Autodesk Inventor part; units mm, degrees
ref_plane "YZ Plane" through (0, 0, 0) normal (1, 0, 0) x (0, 1, 0)
ref_plane "XZ Plane" through (0, 0, 0) normal (0, 1, 0) x (-1, 0, 0)
ref_plane "XY Plane" through (0, 0, 0) normal (0, 0, 1) x (1, 0, 0)
sketch "Skizze1" plane through (0, 0, 0) normal (0, 1, 0) x (-1, 0, 0)
  circle A0 centre (0, 0) radius 9.5
  circle A1 centre (0, 0) radius 11.5
  circle A2 centre (0, 0) radius 8.5
  circle A3 centre (0, 0) radius 3
  circle A4 centre (0, 0) radius 20
  line L0 (10.4225, 4.8601) -> (18.1262, 8.4524)
  line L1 (10.4225, -4.8601) -> (18.1262, -8.4524)
  line L2 (28, 0) -> (-28, 0)
  line L3 (-10.4225, 4.8601) -> (-18.1262, 8.4524)
  line L4 (-10.4225, -4.8601) -> (-18.1262, -8.4524)
  dimension "d0" = 19
  dimension "d1" = 23
  dimension "d2" = 17
  dimension "d3" = 6
  dimension "d8" = 40
  dimension "d10" = 50
extrude "Extrusion1" add sketch "Skizze1" along normal blind 2 contours L2 A2 A0 | L2 A1 A0 | A0 L2 A1 | A0 L2 A2 | L2 A4 L1 A1 | A1 L0 A4 L2 | L2 A3 A2 | A2 L2 A3 | L2 A4 L3 A1 | A1 L4 A4 L2
extrude "Extrusion2" add sketch "Skizze1" against normal blind 10 contours L2 A2 A0 | A0 L2 A2 | L2 A3 A2 | A2 L2 A3
sketch "Skizze2" plane through (0, 2, 0) normal (0, 1, 0) x (1, 0, 0)
  circle A0 centre (0, 0) radius 3
  arc A1 (-18.1262, 8.4524) -> (-18.1262, -8.4524) centre (0, 0) ccw
  line L0 (-2.8868, 5) -> (2.8868, 5)
  line L1 (2.8868, 5) -> (5.7735, 0)
  line L2 (5.7735, 0) -> (2.8868, -5)
  line L3 (2.8868, -5) -> (-2.8868, -5)
  line L4 (-2.8868, -5) -> (-5.7735, 0)
  line L5 (-5.7735, 0) -> (-2.8868, 5)
  dimension "d11" = 10
extrude "Extrusion3" cut sketch "Skizze2" against normal blind 4
properties part number "Unterdruckventil_Gegenhalter"
Verification items for the finished model (mm, model axes). A direction names the side the tool comes from. Give positions to 0.01 mm unless a question says otherwise; leave off trailing zeros. Order: outer loops, then holes, each group sorted by start corner. A loop starts at its lowest first (then second) coordinate and runs counter-clockwise, first axis right, second up. Notation, with made-up numbers: (88, -22.5) -> (142, -22.5) arc R22 cw to (142, -0.5) -> close; hole circle Ø3 at (72.5, -0.5). An arc over 180 degrees is marked (long way). One line per item, written item: value.
(1) Sectioned sample at A-A on x = 0. Record the cut outline in (y, z).
Final values:
outline: (-10, -9.5) -> (0, -9.5) -> (0, -11.5) -> (2, -11.5) -> (2, -5) -> (-2, -5) -> (-2, -3) -> (-10, -3) -> close; (-10, 3) -> (-2, 3) -> (-2, 5) -> (2, 5) -> (2, 11.5) -> (0, 11.5) -> (0, 9.5) -> (-10, 9.5) -> close
(2) Sectioned sample at D-D on z = -3.75. Record the cut outline in (x, y), then the cut area to 3 significant figures.
Final values:
outline: (-19.65, 0) -> (-8.73, 0) -> (-8.73, -10) -> (8.73, -10) -> (8.73, 0) -> (19.65, 0) -> (19.65, 2) -> (3.61, 2) -> (3.61, -2) -> (-3.61, -2) -> (-3.61, 2) -> (-19.65, 2) -> close
area: 224 mm^2
(3) Scan lines: line 1 along Z through (x, y) = (0, -4.5); line 2 along Y through (x, z) = (-5, 8.25); line 3 along Z through (x, y) = (2.5, 1.5). Record each from-to range of solid material in increasing order. Write a range as [from, to].
Final values:
line 1: [-9.5, -3], [3, 9.5]
line 2: [0, 2]
line 3: [-11.22, -5], [5, 11.22]
(4) Tool access check on faces 1 (the face through (0, 0, -10)), 2 (the face through (14.22, 0.99, -6.63)), 3 (the face through (0, 0, 5)). Record the directions out of +Z, -Z, +X, -X, +Y, -Y that give a thin tool (end or side, any length) a straight path to the whole face; none if there is none.
Final values:
face 1: -Y
face 2: -Z, +Y, -Y
face 3: +Y
(5) Gauge pin test, flat ends, axial feed: pin 1 (6 mm diameter, centred on y = 0, z = 8.5, fed in from -X); pin 2 (2 mm diameter, centred on y = -5, z = 4, fed in from +X); pin 3 (1.2 mm diameter, centred on x = 1.5, y = 1, fed in from -Z); pin 4 (2 mm diameter, centred on x = 0.5, y = 0.5, fed in from +Z). Record the tip position at first contact, or that the pin passes through.
Final values:
pin 1: x = -19.23
pin 2: x = 9.01
pin 3: z = -11.46
pin 4: z = 11.5
(6) Sectioned sample at B-B on y = 0.5. Record the cut outline in (x, z), then the cut area to 3 significant figures.
Final values:
outline: (-18.13, -8.45) -> (-10.42, -4.86) arc R11.5 ccw to (10.42, -4.86) -> (18.13, -8.45) arc R20 ccw to (18.13, 8.45) -> (10.42, 4.86) arc R11.5 ccw to (-10.42, 4.86) -> (-18.13, 8.45) arc R20 ccw to start; hole (-5.77, 0) -> (-2.89, -5) -> (2.89, -5) -> (5.77, 0) -> (2.89, 5) -> (-2.89, 5) -> close
area: 563 mm^2
(7) Sectioned sample at C-C on x = -7. Record the cut outline in (y, z).
Final values:
outline: (-10, -6.42) -> (0, -6.42) -> (0, -9.12) -> (2, -9.12) -> (2, 9.12) -> (0, 9.12) -> (0, 6.42) -> (-10, 6.42) -> close
(8) Draft check along Z on faces 4 (the face through (-0.2, 1, -11.5)), 5 (the face through (-4.35, 0.028, -2.465)), 6 (the face through (-14.22, 0.99, 6.63)). Enter one of: pulls with the +Z half, pulls with the -Z half, needs draft (parallel to the pull), parting line crosses it, or undercut.
Final values:
face 4: pulls with the -Z half
face 5: undercut
face 6: pulls with the +Z half
